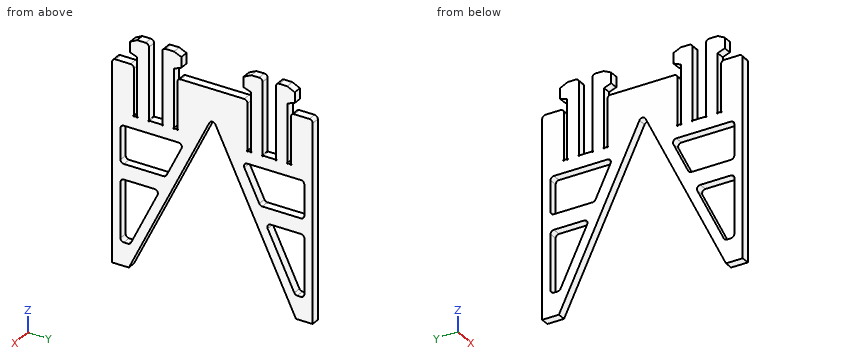
```python
from build123d import *

# Parameters (mm, degrees)
F1_DEPTH = 12.7
F2_R     = 5.08
F3_R     = 5.08
F4_R     = 5.08
F5_R     = 5.08


with BuildPart() as f1:
    # F0 (on Right) → F1 (new body)
    with BuildSketch(Plane.YZ):
        with BuildLine():
            Line((-152.4, -152.4), (-127, -152.4))
            Line((-127, -152.4), (0, 110.3586206897))
            Line((0, 110.3586206897), (-20.32, 152.4))
            Line((-20.32, 152.4), (-53.34, 152.4))
            Line((-53.34, 152.4), (-53.34, 77.216))
            ThreePointArc((-53.34, 77.216), (-52.6215795103, 75.4815795103), (-54.356, 76.2))
            Line((-54.356, 76.2), (-57.4041717125, 76.2))
            ThreePointArc((-57.4041717125, 76.2), (-59.1317859709, 75.4563270968), (-58.42, 77.1973213944))
            Line((-58.42, 77.1973213944), (-58.42, 152.4))
            Line((-58.42, 152.4), (-76.2, 152.4))
            Line((-76.2, 152.4), (-76.2, 77.216))
            ThreePointArc((-76.2, 77.216), (-75.4815795103, 75.4815795103), (-77.216, 76.2))
            Line((-77.216, 76.2), (-95.4923106742, 76.2))
            ThreePointArc((-95.4923106742, 76.2), (-97.2466860912, 75.4733139088), (-96.52, 77.2276893258))
            Line((-96.52, 77.2276893258), (-96.52, 152.4))
            Line((-96.52, 152.4), (-114.3, 152.4))
            Line((-114.3, 152.4), (-114.3, 77.2051736712))
            ThreePointArc((-114.3, 77.2051736712), (-113.5892348808, 75.4892348808), (-115.3051736712, 76.2))
            Line((-115.3051736712, 76.2), (-118.3691862392, 76.2))
            ThreePointArc((-118.3691862392, 76.2), (-120.0947532647, 75.4852467353), (-119.38, 77.2108137608))
            Line((-119.38, 77.2108137608), (-119.38, 152.4))
            Line((-119.38, 152.4), (-152.4, 152.4))
            Line((-152.4, 152.4), (-152.4, -152.4))
        make_face()
        Polygon((-125.2390742302, -117.1909989266), (-139.7, -117.1909989266), (-139.7, -23.267487064), (-79.8427101633, -23.267487064), align=None, mode=Mode.SUBTRACT)
        Polygon((-71.0798129439, 0), (-139.7, 0), (-139.7, 57.1620902733), (-43.4514693118, 57.1620902733), align=None, mode=Mode.SUBTRACT)
        Polygon((-20.32, 152.4), (0, 110.3586206897), (20.32, 152.4), align=None)
        Polygon((-114.3, 165.608), (-114.3, 152.4), (-96.52, 152.4), (-96.52, 191.008), (-114.4882887602, 191.008), (-125.171661377, 185.4585111141), (-125.171661377, 169.4956421852), align=None)
        Polygon((-76.2, 152.4), (-58.42, 152.4), (-58.42, 165.3668519163), (-47.2367718493, 170.141807182), (-47.2367718493, 186.1046761109), (-58.2317112398, 191.008), (-76.2, 191.008), align=None)
        with BuildLine():
            Line((152.4, -152.4), (152.4, 152.4))
            Line((152.4, 152.4), (119.38, 152.4))
            Line((119.38, 152.4), (119.38, 77.2108137608))
            ThreePointArc((119.38, 77.2108137608), (120.0947532647, 75.4852467353), (118.3691862392, 76.2))
            Line((118.3691862392, 76.2), (115.3051736712, 76.2))
            ThreePointArc((115.3051736712, 76.2), (113.5892348808, 75.4892348808), (114.3, 77.2051736712))
            Line((114.3, 77.2051736712), (114.3, 152.4))
            Line((114.3, 152.4), (96.52, 152.4))
            Line((96.52, 152.4), (96.52, 77.2276893258))
            ThreePointArc((96.52, 77.2276893258), (97.2466860912, 75.4733139088), (95.4923106742, 76.2))
            Line((95.4923106742, 76.2), (77.216, 76.2))
            ThreePointArc((77.216, 76.2), (75.4815795103, 75.4815795103), (76.2, 77.216))
            Line((76.2, 77.216), (76.2, 152.4))
            Line((76.2, 152.4), (58.42, 152.4))
            Line((58.42, 152.4), (58.42, 77.1973213944))
            ThreePointArc((58.42, 77.1973213944), (59.1317859709, 75.4563270968), (57.4041717125, 76.2))
            Line((57.4041717125, 76.2), (54.356, 76.2))
            ThreePointArc((54.356, 76.2), (52.6215795103, 75.4815795103), (53.34, 77.216))
            Line((53.34, 77.216), (53.34, 152.4))
            Line((53.34, 152.4), (20.32, 152.4))
            Line((20.32, 152.4), (0, 110.3586206897))
            Line((0, 110.3586206897), (127, -152.4))
            Line((127, -152.4), (152.4, -152.4))
        make_face()
        Polygon((139.7, -117.1909989266), (125.8725191181, -117.1909989266), (80.4761550512, -23.267487064), (139.7, -23.267487064), align=None, mode=Mode.SUBTRACT)
        Polygon((139.7, 0), (72.6210160618, 0), (44.9926724297, 57.1620902733), (139.7, 57.1620902733), align=None, mode=Mode.SUBTRACT)
        Polygon((58.42, 152.4), (76.2, 152.4), (76.2, 166.0996880174), (76.2, 191.1524534295), (59.0350851188, 191.008), (47.548338623, 185.4211749058), (47.548338623, 169.4616637616), (58.42, 165.608), align=None)
        Polygon((96.52, 152.4), (114.3, 152.4), (114.3, 165.608), (125.1717001088, 169.4615544924), (125.1717001088, 185.4210656367), (113.6850067591, 191.008), (96.52, 191.141088813), (96.52, 166.109945806), align=None)
    extrude(amount=F1_DEPTH)

    # F2
    f2_edges = [f1.edges().sort_by_distance(p)[0] for p in [
        (6.35, -139.7, 57.16209),
        (6.35, -43.451469, 57.16209),
        (6.35, -71.079813, 0),
        (6.35, -139.7, 0),
    ]]
    fillet(f2_edges, radius=F2_R)

    # F3
    f3_edges = [f1.edges().sort_by_distance(p)[0] for p in [
        (6.35, -139.7, -23.267487),
        (6.35, -79.84271, -23.267487),
        (6.35, -125.239074, -117.190999),
        (6.35, -139.7, -117.190999),
    ]]
    fillet(f3_edges, radius=F3_R)

    # F4
    f4_edges = [f1.edges().sort_by_distance(p)[0] for p in [
        (6.35, 139.7, 57.16209),
        (6.35, 44.992672, 57.16209),
        (6.35, 72.621016, 0),
        (6.35, 139.7, 0),
        (6.35, 139.7, -23.267487),
        (6.35, 80.476155, -23.267487),
        (6.35, 125.872519, -117.190999),
        (6.35, 139.7, -117.190999),
    ]]
    fillet(f4_edges, radius=F4_R)

    # F5
    f5_edges = [f1.edges().sort_by_distance(p)[0] for p in [
        (6.35, -119.38, 152.4),
        (6.35, -152.4, 152.4),
        (6.35, -53.34, 152.4),
        (6.35, 53.34, 152.4),
        (6.35, 119.38, 152.4),
        (6.35, 152.4, 152.4),
        (6.35, 0, 110.358621),
        (6.35, -96.52, 191.008),
        (6.35, -76.2, 191.008),
        (6.35, 96.52, 191.141089),
        (6.35, 76.2, 191.152453),
    ]]
    fillet(f5_edges, radius=F5_R)


solid = f1.part
```
Can you work these out from the model? Positions are in its coordinate system, mm. Round coordinates to 2 decimals unless told otherwise and drop trailing zeros. Loops run counter-clockwise (first coordinate to the right, second up) from the corner with the lowest first, then second, coordinate; pieces in that order, holes last. Notation, with made-up numbers: M 63,79.25 L 94,79.25 A25 cw 94,107.25 Z; hole C 31,15.25 d6. An arc over 180 degrees is marked long. Answer as a JSON object with one key per item and string values. Group by question number.
Q1. Will these pins go through, and if not, where does the flat tip stop? pin 1 (4 mm diameter, centred on x = 4, z = 151.5, fed in from -Y); pin 2 (6.5 mm diameter, centred on x = 6, y = -133.5, fed in from +Z); pin 3 (1.5 mm diameter, centred on x = 3, y = 78.5, fed in from -Z).
Q2. Imagine slicing it at A-A, the plane z = -85. Please give me the cut outline in (x, y), then the cut area to 3 significant figures.
Q3. Imagine slicing it at B-B, the plane x = 2. Count the separate pieces of the cut face and the enclosed holes in it, then the cut area to 3 significant figures.
Q4. Please list where these lines run through material, in increasing order: L1, parallel to Y at x = 2.25, z = -124; L2, parallel to Y at x = 11, z = 44; L3, parallel to Y at x = 1.5, z = 16.5 (3 decimals).
Findings:
{
 "1": {"pin 1": "stops at y = -151.91", "pin 2": "stops at z = 152.4", "pin 3": "stops at z = -53.61"},
 "2": {"outline": "M 0,-152.4 L 12.7,-152.4 L 12.7,-139.7 L 0,-139.7 Z; M 0,-109.68 L 12.7,-109.68 L 12.7,-94.42 L 0,-94.42 Z; M 0,94.42 L 12.7,94.42 L 12.7,110.31 L 0,110.31 Z; M 0,139.7 L 12.7,139.7 L 12.7,152.4 L 0,152.4 Z", "area": "718 mm2"},
 "3": {"separate pieces": "1", "enclosed holes": "4", "area": "42,300 mm2"},
 "4": {"L1": "y = -152.4 to -113.27, 113.27 to 152.4", "L2": "y = -152.4 to -139.7, -49.81 to -32.07, 32.07 to 51.35, 139.7 to 152.4", "L3": "y = -152.4 to -139.7, -63.105 to -45.365, 45.365 to 64.646, 139.7 to 152.4"}
}
